Verification items for this drawing (mm, ordinates from the low corner). A direction names the side the tool comes from. Coordinates: 2 decimals unless noted, no trailing zeros. Order: outer loops, then holes, each group sorted by start corner. A loop starts at its lowest first (then second) coordinate and runs counter-clockwise, first axis right, second up. Notation, with made-up numbers: M 47.5,-6 L 94.5,-6 A9 cw 94.5,1 Z; hole C -34,0.25 d11. An arc over 180 degrees is marked long. Return JSON: item names as keys, results as strings. Group by question number.
1. Section check D-D, the plane y = 89. Record the cut outline in (x, z), plus the area to 3 significant figures.
2. Section check A-A, the plane y = 29. Record the cut outline in (x, z).
3. Section check B-B, the plane x = 48. Record the cut outline in (y, z).
4. Material ranges on line 1 along Z through (x, y) = (73, 26.5); line 2 along X through (y, z) = (71, 23); line 3 along Z through (x, y) = (45, 76), recorded low to high.
5. Mould release check, pull along X, two halves, no side actions. Record for the marked faces 1, 2, 3 and 4: +X half, -X half, draft (parallel to the pull), parting line (faces both ways), or undercut.
6. Gauge pin test, flat ends, axial feed: pin 1 (3 mm diameter, centred on x = 69, z = 2.5, fed in from -Y); pin 2 (3 mm diameter, centred on x = 2, z = 20, fed in from -Y); pin 3 (12 mm diameter, centred on x = 41, z = 38.5, fed in from -Y). Record the tip position at first contact, or that the pin passes through.
7. Set-up check for the marked faces 5, 6, 7 and 8: record each of +Z, -Z, +X, -X, +Y, -Y from which the full face is reachable in a straight line by a thin tool's end or side.
8. Section check C-C, the plane z = 5. Record the cut outline in (x, y), plus the area to 3 significant figures.
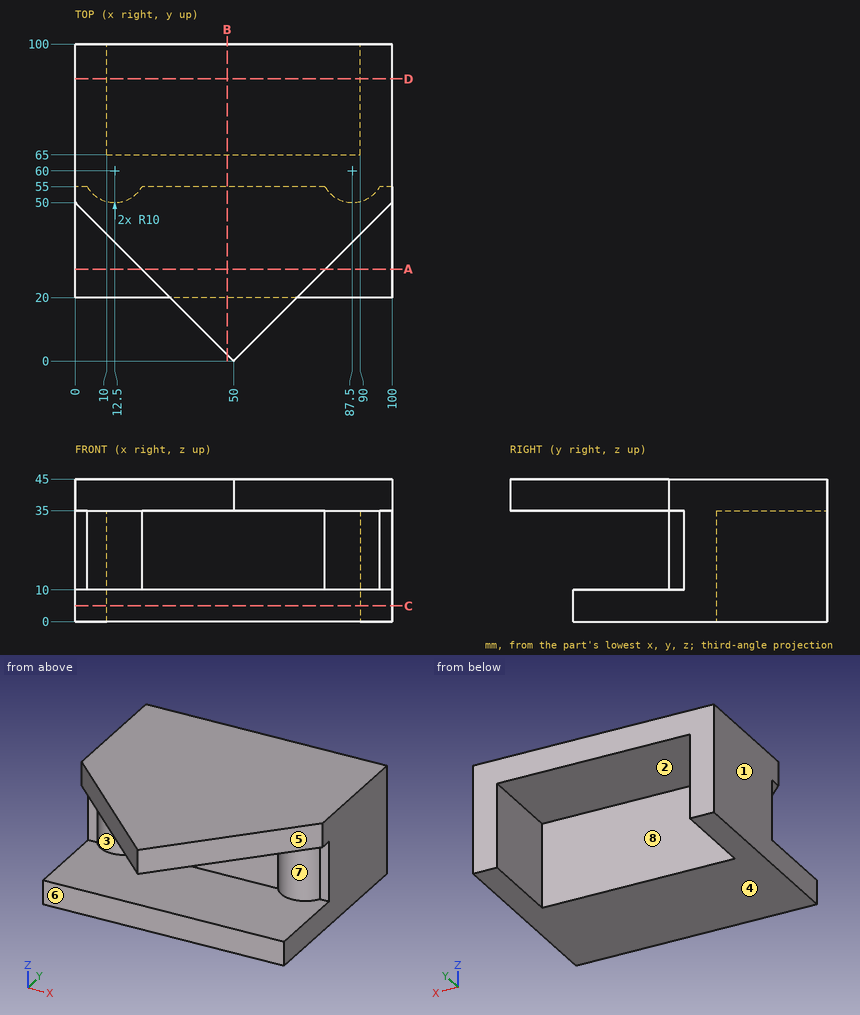
Answers follow:
{
 "1": {"outline": "M 0,0 L 10,0 L 10,35 L 90,35 L 90,0 L 100,0 L 100,45 L 0,45 Z", "area": "1,700 mm^2"},
 "2": {"outline": "M 0,0 L 100,0 L 100,10 L 0,10 Z; M 21,35 L 79,35 L 79,45 L 21,45 Z"},
 "3": {"outline": "M 2,35 L 55,35 L 55,10 L 20,10 L 20,0 L 65,0 L 65,35 L 100,35 L 100,45 L 2,45 Z"},
 "4": {"line 1": "0 to 10, 35 to 45", "line 2": "0 to 10, 90 to 100", "line 3": "35 to 45"},
 "5": {"face 1": "-X half", "face 2": "undercut", "face 3": "undercut", "face 4": "draft"},
 "6": {"pin 1": "y = 20", "pin 2": "y = 55", "pin 3": "y = 3"},
 "7": {"face 5": "+Z, +X, -Y", "face 6": "-Z, +X, -X, -Y", "face 7": "-Y", "face 8": "-Z, +Y"},
 "8": {"outline": "M 0,20 L 100,20 L 100,100 L 90,100 L 90,65 L 10,65 L 10,100 L 0,100 Z", "area": "5,200 mm^2"}
}
